from build123d import *

# Parameters (mm, degrees)
SKETCH_1_R          = 2.05
SKETCH_1_W          = 10
SKETCH_1_H          = 20
EXTRUDE_1_DEPTH     = 5
SKETCH_4_R          = 2.2
CUT_EXTRUDE_1_DEPTH = 222.894677065


with BuildPart() as part:
    # 草圖1 → 填料-伸長1 (new body)
    with BuildSketch(Plane(origin=(0, 0, 0), x_dir=(1, 0, 0), z_dir=(0, 1, 0))):
        with BuildLine():
            Line((193, -80.25), (-193, -80.25))
            ThreePointArc((-193, -80.25), (-206.814373799, 0), (-193, 80.25))
            Line((-193, 80.25), (193, 80.25))
            ThreePointArc((193, 80.25), (206.814373799, 0), (193, -80.25))
        make_face()
        with Locations(Location((0, 71.25, 0), (0, 0, 270))):
            Circle(SKETCH_1_R, mode=Mode.SUBTRACT)
        with Locations(Location((61.70431002, -35.625, 0), (0, 0, 270))):
            Circle(SKETCH_1_R, mode=Mode.SUBTRACT)
        with Locations(Location((-61.70431002, -35.625, 0), (0, 0, 270))):
            Circle(SKETCH_1_R, mode=Mode.SUBTRACT)
        with Locations((178, -25)):
            Rectangle(SKETCH_1_W, SKETCH_1_H, mode=Mode.SUBTRACT)
        with Locations((-178, -25)):
            Rectangle(SKETCH_1_W, SKETCH_1_H, mode=Mode.SUBTRACT)
        with Locations((-178, 25)):
            Rectangle(SKETCH_1_W, SKETCH_1_H, mode=Mode.SUBTRACT)
        with Locations((178, 25)):
            Rectangle(SKETCH_1_W, SKETCH_1_H, mode=Mode.SUBTRACT)
    extrude(amount=EXTRUDE_1_DEPTH)

    # 草圖4 → 除料-伸長1 (cut, through all)
    with BuildSketch(Plane(origin=(0, 5, 0), x_dir=(1, 0, 0), z_dir=(0, 1, 0))):
        with Locations(Location((-138.2, 20, 0), (0, 0, 270))):
            Circle(SKETCH_4_R)
        with Locations(Location((-96.2, 20, 0), (0, 0, 270))):
            Circle(SKETCH_4_R)
        with Locations(Location((-96.2, -20, 0), (0, 0, 270))):
            Circle(SKETCH_4_R)
        with Locations(Location((-138.2, -20, 0), (0, 0, 270))):
            Circle(SKETCH_4_R)
        with Locations(Location((96.2, -20, 0), (0, 0, 90))):
            Circle(SKETCH_4_R)
        with Locations(Location((138.2, -20, 0), (0, 0, 90))):
            Circle(SKETCH_4_R)
        with Locations(Location((96.2, 20, 0), (0, 0, 90))):
            Circle(SKETCH_4_R)
        with Locations(Location((138.2, 20, 0), (0, 0, 90))):
            Circle(SKETCH_4_R)
        with BuildLine():
            Line((-96.9, 63.65), (-93.9, 63.65))
            ThreePointArc((-93.9, 63.65), (-91.4, 61.15), (-93.9, 58.65))
            Line((-93.9, 58.65), (-96.9, 58.65))
            ThreePointArc((-96.9, 58.65), (-99.4, 61.15), (-96.9, 63.65))
        make_face()
        with BuildLine():
            Line((-128.9, 63.65), (-125.9, 63.65))
            ThreePointArc((-125.9, 63.65), (-123.4, 61.15), (-125.9, 58.65))
            Line((-125.9, 58.65), (-128.9, 58.65))
            ThreePointArc((-128.9, 58.65), (-131.4, 61.15), (-128.9, 63.65))
        make_face()
        with BuildLine():
            Line((-96.9, -63.65), (-93.9, -63.65))
            ThreePointArc((-93.9, -63.65), (-91.4, -61.15), (-93.9, -58.65))
            Line((-93.9, -58.65), (-96.9, -58.65))
            ThreePointArc((-96.9, -58.65), (-99.4, -61.15), (-96.9, -63.65))
        make_face()
        with BuildLine():
            Line((-128.9, -63.65), (-125.9, -63.65))
            ThreePointArc((-125.9, -63.65), (-123.4, -61.15), (-125.9, -58.65))
            Line((-125.9, -58.65), (-128.9, -58.65))
            ThreePointArc((-128.9, -58.65), (-131.4, -61.15), (-128.9, -63.65))
        make_face()
        with BuildLine():
            Line((96.9, -63.65), (93.9, -63.65))
            ThreePointArc((93.9, -63.65), (91.4, -61.15), (93.9, -58.65))
            Line((93.9, -58.65), (96.9, -58.65))
            ThreePointArc((96.9, -58.65), (99.4, -61.15), (96.9, -63.65))
        make_face()
        with BuildLine():
            Line((128.9, -63.65), (125.9, -63.65))
            ThreePointArc((125.9, -63.65), (123.4, -61.15), (125.9, -58.65))
            Line((125.9, -58.65), (128.9, -58.65))
            ThreePointArc((128.9, -58.65), (131.4, -61.15), (128.9, -63.65))
        make_face()
        with BuildLine():
            Line((96.9, 63.65), (93.9, 63.65))
            ThreePointArc((93.9, 63.65), (91.4, 61.15), (93.9, 58.65))
            Line((93.9, 58.65), (96.9, 58.65))
            ThreePointArc((96.9, 58.65), (99.4, 61.15), (96.9, 63.65))
        make_face()
        with BuildLine():
            Line((128.9, 63.65), (125.9, 63.65))
            ThreePointArc((125.9, 63.65), (123.4, 61.15), (125.9, 58.65))
            Line((125.9, 58.65), (128.9, 58.65))
            ThreePointArc((128.9, 58.65), (131.4, 61.15), (128.9, 63.65))
        make_face()
    extrude(amount=-CUT_EXTRUDE_1_DEPTH, mode=Mode.SUBTRACT)


solid = part.part
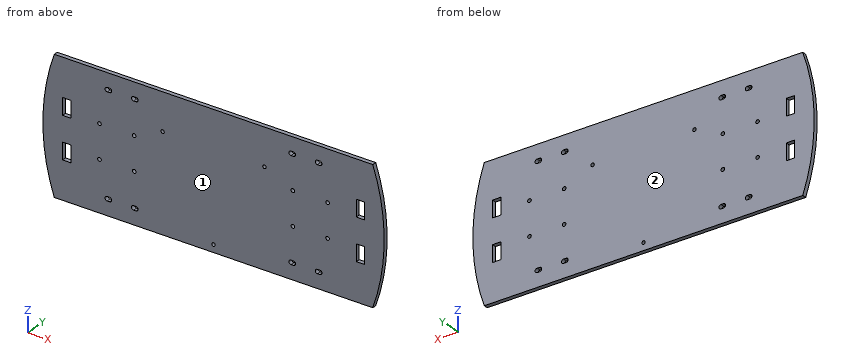
Geometry: final body of the model. Coordinates: model frame, mm. Face numbers are marked on the shaded views. Round coordinates to 2 decimals unless told otherwise and drop trailing zeros. Loops run counter-clockwise (first coordinate to the right, second up) from the corner with the lowest first, then second, coordinate; pieces in that order, holes last. Notation, with made-up numbers: (4, 33.25) - (41, 33.25) arc R26 ccw to (41, 71.25) - close; hole circle Ø1 at (0.5, 1). An arc over 180 degrees is marked (long way). Write each question's results on one line, items separated by ' | '. Start each with the question number.
1) Cut plane A-A on z = 28. Return loops of the section in (x, y).
2) Mould query, pull axis Y, two halves, no side actions, for the marked faces 1 and 2. Classes: released by +Y, released by -Y, zero draft, split by the parting line, or undercut.
3) Line query: probe 1 along Z at (x, y) = (96.2, 3.3); probe 2 along X at (y, z) = (4.7, -33.5); probe 3 along X at (y, z) = (4.1, 73). Output: solid intervals per line, ascending. Write a range as [from, to].
4) First-contact query: P1, Ø2.5, axis at x = -138.2, z = 20, coming from the +Y side; P2, Ø1.5, axis at y = 1, z = 19.5, coming from the -X side; P3, Ø12, axis at x = 132, z = -48, coming from the -Y side; P4, Ø1, axis at y = 2.5, z = -11, coming from the -X side. Flat tips, straight axial feed; report the tip coordinate or a pass-through.
5) Cut plane B-B on z = -27.5. Return loops of the section in (x, y).
6) Cut plane C-C on y = 1.95. Count the separate pieces of the cut face and the enclosed holes in it, then the cut area to 3 significant figures.
Verdict:
1) outline: (-205.18, 0) - (-183, 0) - (-183, 5) - (-205.18, 5) - close; (-173, 0) - (173, 0) - (173, 5) - (-173, 5) - close; (183, 0) - (205.18, 0) - (205.18, 5) - (183, 5) - close
2) face 1: released by -Y | face 2: released by +Y
3) probe 1: z = [-80.25, -63.65], [-58.65, -22.2], [-17.8, 17.8], [22.2, 58.65], [63.65, 80.25] | probe 2: x = [-204.46, -183], [-173, 173], [183, 204.46] | probe 3: x = [-195.44, 195.44]
4) P1: passes through | P2: stops at x = -206.08 | P3: stops at y = 0 | P4: stops at x = -206.58
5) outline: (-205.23, 0) - (-183, 0) - (-183, 5) - (-205.23, 5) - close; (-173, 0) - (173, 0) - (173, 5) - (-173, 5) - close; (183, 0) - (205.23, 0) - (205.23, 5) - (183, 5) - close
6) separate pieces: 1 | enclosed holes: 23 | area: 63,700 mm2
